from build123d import *

# Parameters (mm, degrees)
CYLINDER_R               = 18
CYLINDER_DEPTH           = 30
CYLINDER_PLACEMENT_ANGLE = 120
PAD_DEPTH                = 12
POCKET_DEPTH             = 40.001
SKETCH002_W              = 2.5
SKETCH002_H              = 7.3
POCKET001_DEPTH          = 9


with BuildPart() as cilindro:
    # Cylinder → Cylinder (new body)
    with BuildSketch(Plane.XY):
        Circle(CYLINDER_R)
    extrude(amount=CYLINDER_DEPTH)


with BuildPart() as cilindro_1:
    # Cylinder placement: moved
    add(cilindro.part.moved(Location((0, -5, 29))).rotate(Axis((0, -5, 29), (1, 0, 0)), CYLINDER_PLACEMENT_ANGLE))


with BuildPart() as cut:
    # Sketch → Pad (new body)
    with BuildSketch(Plane.XY):
        Polygon((-20, 12), (20, 12), (20, 0), (10, -15), (-10, -15), (-20, 0), align=None)
    extrude(amount=PAD_DEPTH)

    # Sketch001 (on Face6 of Pad) → Pocket (cut, through all)
    with BuildSketch(Plane(origin=(-20, 0, 0), x_dir=(0, -1, 0), z_dir=(-1, 0, 0))):
        Polygon((0, 12), (15, 5), (15, 12), align=None)
    extrude(amount=-POCKET_DEPTH, mode=Mode.SUBTRACT)

    # Sketch002 (on Face1 of Pocket) → Pocket001 (cut)
    with BuildSketch(Plane(origin=(0, 12, 0), x_dir=(-1, 0, 0), z_dir=(0, 1, 0))):
        with Locations((-14.5, 6)):
            Rectangle(SKETCH002_W, SKETCH002_H)
    pocket001 = extrude(amount=-POCKET001_DEPTH, mode=Mode.SUBTRACT)

    # Mirrored: Pocket001 across Sketch002 V_Axis
    add(pocket001.mirror(Plane(origin=(0, 12, 0), x_dir=(0, 1, 0), z_dir=(-1, 0, 0))), mode=Mode.SUBTRACT)

    # Cut: cut Cilindro
    add(cilindro_1.part, mode=Mode.SUBTRACT)


solid = cut.part
Check sheet for the modelled part. Datum: model origin and axes. Units: mm. A direction names the side the tool comes from. Round coordinates to 2 decimals unless told otherwise and drop trailing zeros. Order: outer loops, then holes, each group sorted by start corner. A loop starts at its lowest first (then second) coordinate and runs counter-clockwise, first axis right, second up.
Q1. Scan lines: L1, parallel to X at y = 10, z = 9; L2, parallel to Z at x = -14.5, y = 8.25; L3, parallel to Z at x = 10, y = -2.75. Record each from-to range of solid material in increasing order.
Filled sheet:
L1: x = -20 to -15.75, -13.25 to 13.25, 15.75 to 20
L2: z = 0 to 2.35, 9.65 to 12
L3: z = 0 to 10.72
Q2. Cross-section at A-A, the plane y = 9.5. Enter the section's corners in (x, z).
Filled sheet:
outline: (-20, 0) - (20, 0) - (20, 12) - (-20, 12) - close; hole (-15.75, 2.35) - (-13.25, 2.35) - (-13.25, 9.65) - (-15.75, 9.65) - close; hole (13.25, 2.35) - (15.75, 2.35) - (15.75, 9.65) - (13.25, 9.65) - close
Q3. Set-up check for faces 4 (the face through (-15.75, 8, 6)), 5 (the face through (0, -1, 0)): record each of +Z, -Z, +X, -X, +Y, -Y from which the full face is reachable in a straight line by a thin tool's end or side.
Filled sheet:
face 4: +Y
face 5: -Z, +X, -X, +Y, -Y
Q4. Depth check by flat-ended pin: P1, Ø1.5, axis at x = 9.5, y = -5.5, coming from the +Z side; P2, Ø1.2, axis at x = -14, z = 6.5, coming from the +Y side. Enter the tip coordinate at first touch or a pass-through.
Filled sheet:
P1: stops at z = 9.78
P2: stops at y = 3
Q5. Cross-section at B-B, the plane z = 1. Enter the section's corners in (x, y).
Filled sheet:
outline: (-20, 0) - (-10, -15) - (10, -15) - (20, 0) - (20, 12) - (-20, 12) - close
Q6. Draft check along Z on faces 1 (the face through (0, 6, 12)), 2 (the face through (15, 8, 9.65)), 3 (the face through (0, -15, 2)). Enter one of: pulls with the +Z half, pulls with the -Z half, needs draft (parallel to the pull), parting line crosses it, or undercut.
Filled sheet:
face 1: pulls with the +Z half
face 2: undercut
face 3: needs draft
Q7. Cross-section at C-C, the plane x = 10.5. Enter the section's corners in (y, z), plus the area to 3 significant figures.
Filled sheet:
outline: (-14.25, 0) - (12, 0) - (12, 12) - (0, 12) - (-14.25, 5.35) - close
area: 268 mm2
Q8. Cross-section at D-D, the plane x = -3. Enter the section's corners in (y, z), plus the area to 3 significant figures.
Filled sheet:
outline: (-15, 0) - (12, 0) - (12, 12) - (1.05, 12) - (-15, 2.73) - close
area: 250 mm2
